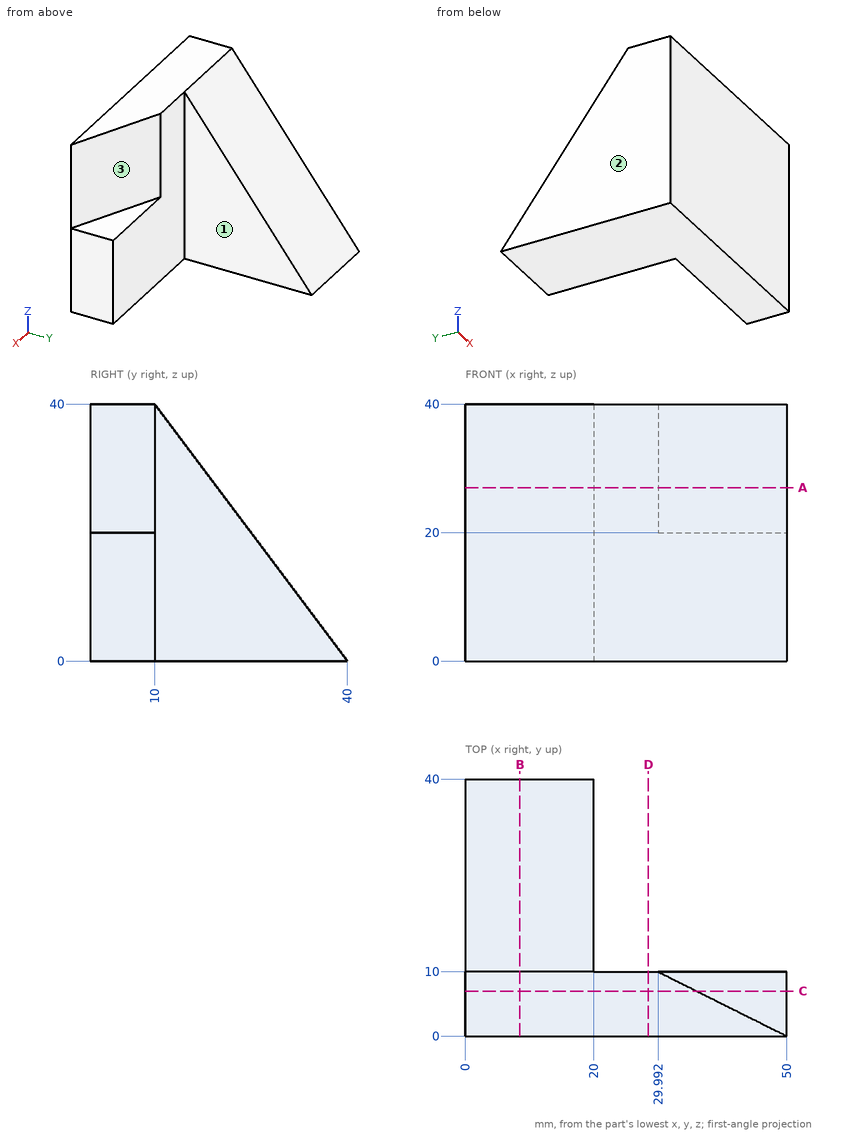
Can you work these out from the drawing? Everything is in mm from the part's minimum corner. A direction names the side the tool comes from. Give positions to 0.01 mm unless a question says otherwise; leave off trailing zeros. Order: outer loops, then holes, each group sorted by start corner. A loop starts at its lowest first (then second) coordinate and runs counter-clockwise, first axis right, second up.
1. Will these pins go through, and if not, where does the flat tip stop? P1, Ø15, axis at x = 30, z = 10, coming from the +Y side; P2, Ø3, axis at x = 11.5, z = 34.5, coming from the -Y side; P3, Ø10, axis at y = 30.5, z = 11.5, coming from the +X side; P4, Ø6, axis at x = 6.5, z = 15, coming from the +Y side.
2. Suppose I cut it at A-A (z = 27). List the corners of the cut face in (x, y) for me.
3. Suppose I cut it at B-B (x = 8.5). List the corners of the cut face in (y, z) for me.
4. Suppose I cut it at C-C (y = 7). List the corners of the cut face in (x, z) for me (1 decimal), plus the area to 3 significant figures.
5. I need wall thicknesses on L1, parallel to Y at x = 30, z = 10.5; L2, parallel to X at y = 24, z = 7.5; L3, parallel to Y at x = 43, z = 37. Which ranges of each line are inside material? Lowest first, please.
6. Suppose I cut it at D-D (x = 28.5). List the corners of the cut face in (y, z) for me, plus the area to 3 significant figures.
7. For the marked faces 1, 2 and 3, which set-ups out of +Z, -Z, +X, -X, +Y, -Y let a thin tool reach every point of the face, with its end or its side?
Solved:
1. P1: stops at y = 10
1. P2: stops at y = 0
1. P3: stops at x = 20
1. P4: stops at y = 31
2. outline: (0, 0) - (50, 0) - (29.99, 10) - (20, 10) - (20, 19.75) - (0, 19.75) - close
3. outline: (0, 0) - (40, 0) - (10, 40) - (0, 40) - close
4. outline: (0, 0) - (50, 0) - (50, 20) - (36, 20) - (36, 40) - (0, 40) - close
4. area: 1,720 mm2
5. L1: y = 0 to 10
5. L2: x = 0 to 20
5. L3: y = 0 to 3.5
6. outline: (0, 0) - (10, 0) - (10, 40) - (0, 40) - close
6. area: 400 mm2
7. face 1: +Z, -Z, +X, +Y
7. face 2: +Z, -Z, -X, +Y, -Y
7. face 3: +Z, +X, +Y
